```python
from build123d import *

# Parameters (mm, degrees)
SKETCH1_W             = 165.1
SKETCH1_H             = 12.7
BOSS_EXTRUDE1_DEPTH   = 6.35
SKETCH2_W             = 38.1
SKETCH2_H             = 3.81
CUT_EXTRUDE1_DEPTH    = 84.762252835
F_6_CLEARANCE_HOLE1_D = 3.7973
SKETCH6_W             = 9.525
SKETCH6_H             = 19.05
BOSS_EXTRUDE2_DEPTH   = 12.7
F_4_40_TAPPED_HOLE1_D = 2.2606


with BuildPart() as part:
    # Sketch1 → Boss-Extrude1 (new body)
    with BuildSketch(Plane(origin=(0, 0, 0), x_dir=(1, 0, 0), z_dir=(0, 1, 0))):
        Rectangle(SKETCH1_W, SKETCH1_H)
    extrude(amount=BOSS_EXTRUDE1_DEPTH)

    # Sketch2 → Cut-Extrude1 (cut, through all)
    with BuildSketch(Plane.XY.offset(6.35)):
        with Locations((-63.5, 4.445)):
            Rectangle(SKETCH2_W, SKETCH2_H)
    cut_extrude1 = extrude(amount=-CUT_EXTRUDE1_DEPTH, mode=Mode.SUBTRACT)

    # #6 Clearance Hole1 (through all)
    with Locations(Plane(origin=(0, 0, 0), x_dir=(-1, 0, 0), z_dir=(0, -1, 0))):
        with Locations((50.8, 0), (76.2, 0)):
            f_6_clearance_hole1 = Hole(F_6_CLEARANCE_HOLE1_D / 2)

    # Mirror1: Cut-Extrude1, #6 Clearance Hole1 across plane
    add(cut_extrude1.mirror(Plane(origin=(0, 0, 0), x_dir=(0, 0, 1), z_dir=(1, 0, 0))), mode=Mode.SUBTRACT)
    add(f_6_clearance_hole1.mirror(Plane(origin=(0, 0, 0), x_dir=(0, 0, 1), z_dir=(1, 0, 0))), mode=Mode.SUBTRACT)

    # Sketch6 → Boss-Extrude2 (add)
    with BuildSketch(Plane.XY.offset(6.35)):
        with Locations((7.9375, -9.525)):
            Rectangle(SKETCH6_W, SKETCH6_H)
    extrude(amount=-BOSS_EXTRUDE2_DEPTH)

    # #4-40 Tapped Hole1 (through all)
    with Locations(Plane(origin=(12.7, 0, 0), x_dir=(0, 0, -1), z_dir=(1, 0, 0))):
        with Locations((0, -9.525)):
            Hole(F_4_40_TAPPED_HOLE1_D / 2)


solid = part.part
```
CAD build for the part. Positions are in the model's coordinates, mm. A direction names the side the tool comes from. Round coordinates to 2 decimals unless told otherwise and drop trailing zeros. Write each loop counter-clockwise with the first axis right and the second up, starting at its lowest first coordinate (ties: lowest second). Pieces come first, ordered by that corner, then holes. Notation, with made-up numbers: (38, 16.5) -> (90, 16.5) arc R15 ccw to (90, 41.5) -> close; hole circle Ø6 at (-11, 46.5). An arc over 180 degrees is marked (long way). Answer in a Markdown table with one row per item. Add a question column.
Item 1: Saw through at A-A, the plane x = -76.2. Write the cut outline in (y, z).
Item 2: Drill centre lines: line 1 (Z direction, x = -50.8, y = 0.9); line 2 (X direction, y = 0.25, z = -1.25); line 3 (X direction, y = -12, z = 4.5) (3 decimals). Where is each one in solid material? Low to high. Write a range as from..to.
Item 3: Saw through at D-D, the plane x = -32. Write the cut outline in (y, z), then the cut area to 3 significant figures.
Item 4: Which spindle directions (+Z, -Z, +X, -X, +Y, -Y) get a long thin tool onto all of the face, cutting with end or side? Do faces 4 (the face through (-64, 2.54, 0)), 5 (the face through (64, 2.54, 0)), 6 (the face through (47, 0, 0)). Say none if no direction does.
Item 5: Saw through at C-C, the plane y = 4.75. Write the cut outline in (x, z), then the cut area to 3 significant figures.
Item 6: Drop flat-ended pins along their axis: pin 1 Ø2.5 at (x, z) = (50.8, 0) entering from -Y; pin 2 Ø4.5 at (x, z) = (-50.8, 0) entering from -Y; pin 3 Ø6.5 at (x, z) = (64.5, 2) entering from +Y; pin 4 Ø1.9 at (y, z) = (5, -1.5) entering from +X. Give the stop position or say it passes through.
Item 7: Mould opens along Z. For faces 1 (the face through (0, 1, -6.35)), 2 (the face through (-82.55, 1, 0)), 3 (the face through (74.4, 1.3, -0.6)) say: pulls with the +Z half, pulls with the -Z half, needs draft (parallel to the pull), parting line crosses it, or undercut.
Item 8: Saw through at B-B, the plane z = -3.5. Write the cut outline in (x, y) (3 decimals).
Findings below:
| question | item | result |
|---|---|---|
| 1 | outline | (0, -6.35) -> (2.54, -6.35) -> (2.54, -1.9) -> (0, -1.9) -> close; (0, 1.9) -> (2.54, 1.9) -> (2.54, 6.35) -> (0, 6.35) -> close |
| 2 | line 1 | z = -6.35..-1.9, 1.9..6.35 |
| 2 | line 2 | x = -82.55..-77.63, -74.77..-52.23, -49.37..49.37, 52.23..74.77, 77.63..82.55 |
| 2 | line 3 | x = 3.175..12.7 |
| 3 | outline | (0, -6.35) -> (6.35, -6.35) -> (6.35, 6.35) -> (0, 6.35) -> close |
| 3 | area | 80.6 mm^2 |
| 4 | face 4 | +Z, -Z, -X, +Y |
| 4 | face 5 | +Z, -Z, +X, +Y |
| 4 | face 6 | +Z, -Z, +X, -Y |
| 5 | outline | (-44.45, -6.35) -> (44.45, -6.35) -> (44.45, 6.35) -> (-44.45, 6.35) -> close |
| 5 | area | 1,130 mm^2 |
| 6 | pin 1 | passes through |
| 6 | pin 2 | stops at y = 0 |
| 6 | pin 3 | stops at y = 2.54 |
| 6 | pin 4 | stops at x = 44.45 |
| 7 | face 1 | pulls with the -Z half |
| 7 | face 2 | needs draft |
| 7 | face 3 | undercut |
| 8 | outline | (-82.55, 0) -> (3.175, 0) -> (3.175, -19.05) -> (12.7, -19.05) -> (12.7, 0) -> (82.55, 0) -> (82.55, 2.54) -> (44.45, 2.54) -> (44.45, 6.35) -> (-44.45, 6.35) -> (-44.45, 2.54) -> (-82.55, 2.54) -> close |
